Autodesk Inventor part; units mm, degrees
ref_plane "YZ Plane" through (0, 0, 0) normal (1, 0, 0) x (0, 1, 0)
ref_plane "XZ Plane" through (0, 0, 0) normal (0, 1, 0) x (-1, 0, 0)
ref_plane "XY Plane" through (0, 0, 0) normal (0, 0, 1) x (1, 0, 0)
sketch "Sketch1" plane through (0, 0, 0) normal (0, 1, 0) x (-1, 0, 0)
  circle A0 centre (0, 0) radius 9.5
  dimension "d0" = 19
extrude "Extrusion1" add sketch "Sketch1" along normal mid plane 25
sketch "Sketch2" plane through (0, 0, 0) normal (0, 1, 0) x (-1, 0, 0)
  circle A0 centre (0, 0) radius 4
  circle A1 centre (0, 0) radius 2.5
  dimension "d3" = 8
  dimension "d4" = 5
extrude "Extrusion2" cut sketch "Sketch2" against normal blind 25 contours A0 | A1
extrude "Extrusion3" cut sketch "Sketch2" along normal blind 25 contours A1
fillet "Fillet1" radius 0.5 4 edges at (9.5, 12.5, 0) (9.5, -12.5, 0) (2.5, 12.5, 0) (4, -12.5, 0)
properties part number "Flx_Al_Coupling(5_8mm)"
CAD build for the part. Positions are in the model's coordinates, mm. A direction names the side the tool comes from. Round coordinates to 2 decimals unless told otherwise and drop trailing zeros. Write each loop counter-clockwise with the first axis right and the second up, starting at its lowest first coordinate (ties: lowest second). Pieces come first, ordered by that corner, then holes. Notation, with made-up numbers: (-32, 49.25) -> (-27, 49.25) arc R10 ccw to (-27, 68.25) -> close; hole circle Ø4 at (-5.5, 29). An arc over 180 degrees is marked (long way). Answer in a Markdown table with one row per item. Add a question column.
Item 1: Saw through at B-B, the plane x = 0. Write the cut outline in (y, z), then the cut area to 3 significant figures.
Item 2: Saw through at A-A, the plane z = 0. Write the cut outline in (x, y).
Item 3: Which spindle directions (+Z, -Z, +X, -X, +Y, -Y) get a long thin tool onto all of the face, cutting with end or side? Do faces 5 (the face through (0.867, -5.916, -3.905)), 6 (the face through (-4, -12.5, -4)). Say none if no direction does.
Item 4: Drill centre lines: line 1 (Z direction, x = 0, y = 3); line 2 (Z direction, x = -0.25, y = -4.25). Where is each one in solid material? Low to high. Write a range as from..to.
Item 5: Mould opens along Z. For faces 1 (the face through (0, 12.5, -4)), 2 (the face through (-4.38, -0.17, 8.43)), 3 (the face through (-2, 0, 2)), 4 (the face through (0.54, 5.92, 2.44)) say: pulls with the +Z half, pulls with the -Z half, needs draft (parallel to the pull), parting line crosses it, or undercut.
Item 6: Saw through at D-D, the plane y = -6.5. Write the cut outline in (x, z).
Item 7: Saw through at C-C, the plane y = 11.25. Write the cut outline in (x, z), then the cut area to 3 significant figures.
Item 8: Drop flat-ended pins along their axis: pin 1 Ø10 at (y, z) = (5.5, -6.5) entering from -X; pin 2 Ø5 at (x, y) = (3, -5) entering from +Z. Give the stop position or say it passes through.
Findings below:
| question | item | result |
|---|---|---|
| 1 | outline | (-12.5, -9) arc R0.5 ccw to (-12, -9.5) -> (12, -9.5) arc R0.5 ccw to (12.5, -9) -> (12.5, -3) arc R0.5 ccw to (12, -2.5) -> (0, -2.5) -> (0, -4) -> (-12, -4) arc R0.5 ccw to (-12.5, -4.5) -> close; (-12.5, 4.5) arc R0.5 ccw to (-12, 4) -> (0, 4) -> (0, 2.5) -> (12, 2.5) arc R0.5 ccw to (12.5, 3) -> (12.5, 9) arc R0.5 ccw to (12, 9.5) -> (-12, 9.5) arc R0.5 ccw to (-12.5, 9) -> close |
| 1 | area | 312 mm^2 |
| 2 | outline | (-9.5, -12) arc R0.5 ccw to (-9, -12.5) -> (-4.5, -12.5) arc R0.5 ccw to (-4, -12) -> (-4, 0) -> (-2.5, 0) -> (-2.5, 12) arc R0.5 ccw to (-3, 12.5) -> (-9, 12.5) arc R0.5 ccw to (-9.5, 12) -> close; (2.5, 0) -> (4, 0) -> (4, -12) arc R0.5 ccw to (4.5, -12.5) -> (9, -12.5) arc R0.5 ccw to (9.5, -12) -> (9.5, 12) arc R0.5 ccw to (9, 12.5) -> (3, 12.5) arc R0.5 ccw to (2.5, 12) -> close |
| 3 | face 5 | -Y |
| 3 | face 6 | +Z, -Z, +X, -X, -Y |
| 4 | line 1 | z = -9.5..-2.5, 2.5..9.5 |
| 4 | line 2 | z = -9.5..-3.99, 3.99..9.5 |
| 5 | face 1 | needs draft |
| 5 | face 2 | parting line crosses it |
| 5 | face 3 | undercut |
| 5 | face 4 | undercut |
| 6 | outline | circle Ø19 at (0, 0); hole circle Ø8 at (0, 0) |
| 7 | outline | circle Ø19 at (0, 0); hole circle Ø5 at (0, 0) |
| 7 | area | 264 mm^2 |
| 8 | pin 1 | stops at x = -9.38 |
| 8 | pin 2 | stops at z = 9.49 |
